from build123d import *

# Parameters (mm, degrees)
BOSS_EXTRUDE1_DEPTH = 1
SKETCH2_RX          = 1.25
SKETCH2_RY          = 1
CUT_EXTRUDE1_DEPTH  = 15.62450684
BOSS_EXTRUDE2_DEPTH = 0.95
BOSS_EXTRUDE3_DEPTH = 2.1
SKETCH7_W           = 8.190854722
SKETCH7_H           = 2.464294839
BOSS_EXTRUDE4_DEPTH = 4.2
SKETCH8_W           = 4.413735787
SKETCH8_H           = 4.058267134
BOSS_EXTRUDE5_DEPTH = 0.75


with BuildPart() as part:
    # Sketch1 → Boss-Extrude1 (new body)
    with BuildSketch(Plane.XY):
        Polygon((-2.780385667, 3.527721413), (7.219614333, 3.527721413), (7.219614333, 0.277721413), (12.219614333, 0.277721413), (12.219614333, -4.722278587), (7.383278363, -4.722278587), (7.383278363, -7.972278587), (-2.616721637, -7.972278587), (-2.616721637, -4.722278587), (-7.780385667, -4.722278587), (-7.780385667, 0.277721413), (-2.780385667, 0.277721413), align=None)
    extrude(amount=BOSS_EXTRUDE1_DEPTH)

    # Sketch2 → Cut-Extrude1 (cut, through all)
    with BuildSketch(Plane.XY.offset(1)):
        with Locations((9.935757543, -2.200550618)):
            Ellipse(SKETCH2_RX, SKETCH2_RY)
        with Locations(Location((-5.164242457, -2.289417781), (0, 0, 0))):
            Ellipse(SKETCH2_RX, SKETCH2_RY)
    extrude(amount=-CUT_EXTRUDE1_DEPTH, mode=Mode.SUBTRACT)

    # Sketch5 → Boss-Extrude2 (add)
    with BuildSketch(Plane(origin=(0, 0, 0), x_dir=(-1, 0, 0), z_dir=(0, 0, -1))):
        with BuildLine():
            Line((-5.285531474, 1.157258951), (0.514468526, 1.157258951))
            ThreePointArc((0.514468526, 1.157258951), (3.914468526, -2.242741049), (0.514468526, -5.642741049))
            Line((0.514468526, -5.642741049), (-5.285531474, -5.642741049))
            ThreePointArc((-5.285531474, -5.642741049), (-8.685531474, -2.242741049), (-5.285531474, 1.157258951))
        make_face()
    extrude(amount=BOSS_EXTRUDE2_DEPTH)

    # Sketch6 → Boss-Extrude3 (add)
    with BuildSketch(Plane(origin=(0, 0, -0.95), x_dir=(-1, 0, 0), z_dir=(0, 0, -1))):
        with BuildLine():
            Line((-5.063363565, 0.222790462), (0.505645348, 0.222790462))
            ThreePointArc((0.505645348, 0.222790462), (3.005645348, -2.277209538), (0.505645348, -4.777209538))
            Line((0.505645348, -4.777209538), (-5.063363565, -4.777209538))
            ThreePointArc((-5.063363565, -4.777209538), (-7.563363565, -2.277209538), (-5.063363565, 0.222790462))
        make_face()
    extrude(amount=BOSS_EXTRUDE3_DEPTH)

    # Sketch7 → Boss-Extrude4 (add)
    with BuildSketch(Plane.XY.offset(1)):
        with Locations((2.345641724, -6.512937551)):
            Rectangle(SKETCH7_W, SKETCH7_H)
    extrude(amount=BOSS_EXTRUDE4_DEPTH)

    # Sketch8 → Boss-Extrude5 (add)
    with BuildSketch(Plane.XY.offset(1)):
        with Locations((0.264536736, -0.348662557)):
            Rectangle(SKETCH8_W, SKETCH8_H)
    extrude(amount=BOSS_EXTRUDE5_DEPTH)


solid = part.part
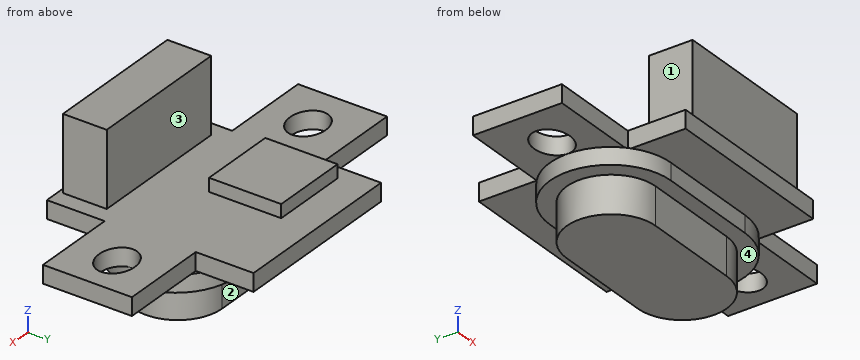
Work out the finished part from the listing and answer in its coordinate system (mm). Face numbers are marked on the shaded views. A direction names the side the tool comes from. Coordinates: 2 decimals unless noted, no trailing zeros. Write each loop counter-clockwise with the first axis right and the second up, starting at its lowest first coordinate (ties: lowest second). Pieces come first, ordered by that corner, then holes. Notation, with made-up numbers: M -38.5,-39.75 L 8.5,-39.75 A30 cw 8.5,-8.75 Z; hole C 38.5,51.5 d10. An arc over 180 degrees is marked long. Answer as CSV lines item,"result". Start each with the question number.
Item 1: Section B-B on y = -6.5 is taken. Write down the section's boundary in (x, z), and give its area (3 significant figures).
Item 2: Section A-A on z = 1.5 is taken. Write down the section's boundary in (x, y).
Item 3: Section C-C on x = 8 is taken. Write down the section's boundary in (y, z).
Item 4: A tool of negligible diameter and unlimited length cuts with its end or side. For the marked faces 1, 2, 3 and 4, from which of +Z, -Z, +X, -X, +Y, -Y can it reach the whole face along a straight path? Write none if from no direction.
Item 5: Section D-D on z = -0.75 is taken. Write down the section's boundary in (x, y), and give its area (3 significant figures).
Item 6: Consider L1, parallel to Z at x = 7.25, y = -4.5; L2, parallel to X at y = -7, z = 2.5; L3, parallel to Y at x = 1, z = -0.75. Determine where each line is inside the solid, lowest interval first.
Item 7: Flat-ended cylindrical pins translate along their axes: P1, Ø1.2, axis at y = -6.5, z = 2.5, coming from the +X side; P2, Ø2, axis at x = 1, y = -0.5, coming from the +Z side; P3, Ø1.5, axis at y = -2, z = 3, coming from the +X side; P4, Ø0.8, axis at x = 2.5, z = -0.5, coming from the -Y side. Find the tip coordinate at first contact, or state that the pin passes through.
Checks:
1,outline,"M -2.62,0 L 7.38,0 L 7.38,1 L 6.44,1 L 6.44,5.2 L -1.75,5.2 L -1.75,1 L -2.62,1 Z"
1,area,"44.4 mm²"
2,outline,"M -1.94,-2.38 L 2.47,-2.38 L 2.47,1.68 L -1.94,1.68 Z; M -1.75,-7.75 L 6.44,-7.75 L 6.44,-5.28 L -1.75,-5.28 Z"
3,outline,"M -4.72,0 L -4.29,0 L -4.29,-0.95 L -0.2,-0.95 L -0.2,0 L 0.28,0 L 0.28,1 L -4.72,1 Z"
4,face 1,"+Z, -X, -Y"
4,face 2,"-Z, +X, -X, +Y"
4,face 3,"+Z, +X, -X"
4,face 4,"-Z"
5,outline,"M -0.51,-5.64 L 5.29,-5.64 A3.4 ccw 5.29,1.16 L -0.51,1.16 A3.4 ccw Z"
5,area,"75.8 mm²"
6,L1,"z = -0.95 to 1"
6,L2,"x = -1.75 to 6.44"
6,L3,"y = -5.64 to 1.16"
7,P1,"stops at x = 6.44"
7,P2,"stops at z = 1.75"
7,P3,"passes through"
7,P4,"stops at y = -5.64"
